Input: part model. Units: mm. Frame: model coordinates. Face numbers are marked on the shaded views. A direction names the side the tool comes from. Round coordinates to 2 decimals unless told otherwise and drop trailing zeros. Loops run counter-clockwise (first coordinate to the right, second up) from the corner with the lowest first, then second, coordinate; pieces in that order, holes last.
1) First-contact query: pin 1 (8 mm diameter, centred on x = 23.5, y = 57, fed in from -Z); pin 2 (6 mm diameter, centred on x = 0, y = 0, fed in from +Z); pin 3 (6 mm diameter, centred on x = -25, z = -2, fed in from -Y). Flat tips, straight axial feed; report the tip coordinate or a pass-through.
2) Section B-B, the plane x = 60. Return loops of the section in (y, z).
3) Section A-A, the plane z = -7.5. Return loops of the section in (x, y) (3 decimals), and give its area (3 significant figures).
4) Section D-D, the plane x = -29. Return loops of the section in (y, z), and give its area (3 significant figures).
5) Ray query, line 1 along Y through (x, z) = (0, -3) (3 decimals); line 2 along Y through (x, z) = (0, 28.5); line 3 along X through (y, z) = (42.5, 25). Return the intervals inside material, ascending.
6) Section C-C, the plane y = -66. Return loops of the section in (x, z).
7) Access query for the marked faces 1, 2 and 3. Directions: +Z, -Z, +X, -X, +Y, -Y. A direction counts if a zero-diameter tool reaches every point of the face in a straight line with its end or side. Return the directions, or none.
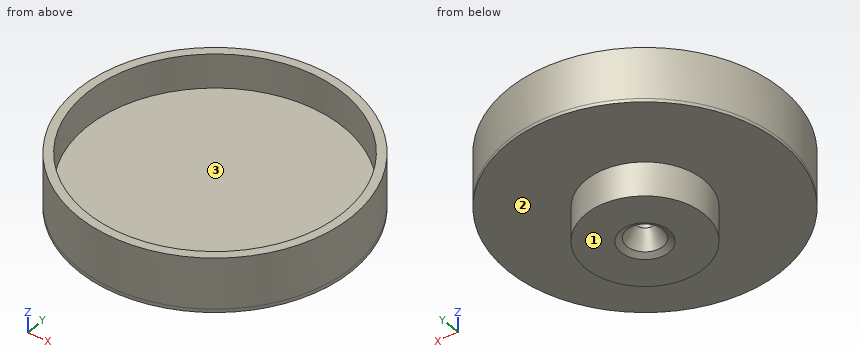
from build123d import *

# Parameters (mm, degrees)
SZKIC1_R                    = 80
DODANIE_WYCI_GNI_CIE1_DEPTH = 30
SZKIC2_R                    = 75
WYTNIJ_WYCI_GNI_CIE2_DEPTH  = 20
DODANIE_WYCI_GNI_CIE2_START = 22
SZKIC20_R                   = 80
DODANIE_WYCI_GNI_CIE2_DEPTH = 22
SZKIC22_R                   = 80
SZKIC22_R_2                 = 34.425
WYTNIJ_WYCI_GNI_CIE3_DEPTH  = 20


with BuildPart() as part:
    # Szkic1 → Dodanie-wyciągnięcie1 (new body)
    with BuildSketch(Plane.XY):
        Circle(SZKIC1_R)
    extrude(amount=DODANIE_WYCI_GNI_CIE1_DEPTH)

    # Szkic2 → Wytnij-wyciągnięcie2 (cut)
    with BuildSketch(Plane.XY.offset(30)):
        Circle(SZKIC2_R)
    extrude(amount=-WYTNIJ_WYCI_GNI_CIE2_DEPTH, mode=Mode.SUBTRACT)

    # Szkic20 → Dodanie-wyciągnięcie2 (add)
    with BuildSketch(Plane(origin=(0, 0, 0), x_dir=(-1, 0, 0), z_dir=(0, 0, -1)).offset(DODANIE_WYCI_GNI_CIE2_START)):
        Circle(SZKIC20_R)
    extrude(amount=-DODANIE_WYCI_GNI_CIE2_DEPTH)

    # Szkic21 → Wycięcie-obrót1 (revolve, cut)
    with BuildSketch(Plane(origin=(0, 0, 0), x_dir=(1, 0, 0), z_dir=(0, 1, 0))):
        Polygon((0, 22), (0, -7.46), (-5, -2.46), (-5, 10.34), (-10.600297611, 20.04), (-13.995117194, 22), align=None)
    revolve(axis=Axis((0, 0, 0), (0, 0, 1)), mode=Mode.SUBTRACT)

    # Szkic22 → Wytnij-wyciągnięcie3 (cut)
    with BuildSketch(Plane(origin=(0, 0, -22), x_dir=(-1, 0, 0), z_dir=(0, 0, -1))):
        Circle(SZKIC22_R)
        Circle(SZKIC22_R_2, mode=Mode.SUBTRACT)
    extrude(amount=-WYTNIJ_WYCI_GNI_CIE3_DEPTH, mode=Mode.SUBTRACT)


solid = part.part
Final values:
1. pin 1: stops at z = -2
1. pin 2: stops at z = 10
1. pin 3: stops at y = -76.92
2. outline: (-52.92, -2) - (52.92, -2) - (52.92, 30) - (45, 30) - (45, 10) - (-45, 10) - (-45, 30) - (-52.92, 30) - close
3. outline: circle Ø68.85 at (0, 0); hole circle Ø10 at (0, 0)
3. area: 3,640 mm2
4. outline: (-74.56, -2) - (-18.55, -2) - (-18.55, -22) - (18.55, -22) - (18.55, -2) - (74.56, -2) - (74.56, 30) - (69.17, 30) - (69.17, 10) - (-69.17, 10) - (-69.17, 30) - (-74.56, 30) - close
4. area: 2,750 mm2
5. line 1: y = -34.425 to -5, 5 to 34.425
5. line 2: y = -80 to -75, 75 to 80
5. line 3: x = -67.78 to -61.8, 61.8 to 67.78
6. outline: (-45.21, -2) - (45.21, -2) - (45.21, 30) - (35.62, 30) - (35.62, 10) - (-35.62, 10) - (-35.62, 30) - (-45.21, 30) - close
7. face 1: -Z, +X, -X, +Y, -Y
7. face 2: -Z
7. face 3: +Z
